The model under review builds one solid part; all positions refer to its coordinate system, in mm. Face numbers are marked on the shaded views. A direction names the side the tool comes from. Round coordinates to 2 decimals unless told otherwise and drop trailing zeros. Loops run counter-clockwise (first coordinate to the right, second up) from the corner with the lowest first, then second, coordinate; pieces in that order, holes last. Notation, with made-up numbers: M 24,2.25 L 51,2.25 A33 cw 51,31.25 Z; hole C 36.25,30 d9. An arc over 180 degrees is marked long. Use a Markdown table: item, result. Add a question column.
```python
from build123d import *

# Parameters (mm, degrees)
SKETCH5_W           = 60
SKETCH5_H           = 55
BOSS_EXTRUDE4_DEPTH = 20
SKETCH6_W           = 55
SKETCH6_H           = 50
CUT_EXTRUDE2_DEPTH  = 17.5
FILLET1_R           = 5
SKETCH8_W           = 45
SKETCH8_H           = 45
BOSS_EXTRUDE5_DEPTH = 5
CUT_EXTRUDE4_REACH  = 49.762
SKETCH9_W           = 15
SKETCH9_H           = 20
CUT_EXTRUDE5_REACH  = 68.802
SKETCH11_W          = 10
SKETCH11_H          = 4


with BuildPart() as part:
    # Sketch5 → Boss-Extrude4 (new body)
    with BuildSketch(Plane(origin=(0, 0, 0), x_dir=(1, 0, 0), z_dir=(0, 1, 0))):
        Rectangle(SKETCH5_W, SKETCH5_H)
    extrude(amount=BOSS_EXTRUDE4_DEPTH)

    # Sketch6 → Cut-Extrude2 (cut)
    with BuildSketch(Plane(origin=(0, 20, 0), x_dir=(1, 0, 0), z_dir=(0, 1, 0))):
        Rectangle(SKETCH6_W, SKETCH6_H)
    extrude(amount=-CUT_EXTRUDE2_DEPTH, mode=Mode.SUBTRACT)

    # Fillet1
    fillet1_edges = [part.edges().sort_by_distance(p)[0] for p in [
        (-30, 10, -27.5),
        (30, 10, -27.5),
        (30, 10, 27.5),
        (-30, 10, 27.5),
    ]]
    fillet(fillet1_edges, radius=FILLET1_R)

    # Sketch8 → Boss-Extrude5 (add)
    with BuildSketch(Plane.XZ):
        Rectangle(SKETCH8_W, SKETCH8_H)
    extrude(amount=BOSS_EXTRUDE5_DEPTH)

    # Sketch9 → Cut-Extrude4 (cut, up to next)
    with BuildSketch(Plane.XZ.offset(5), mode=Mode.PRIVATE) as cut_extrude4_sk1:
        with Locations((-12.5, 10)):
            Rectangle(SKETCH9_W, SKETCH9_H)
    cut_extrude4_tool1 = extrude(cut_extrude4_sk1.sketch, amount=-CUT_EXTRUDE4_REACH, mode=Mode.PRIVATE) & part.part
    add(cut_extrude4_tool1.solids().sort_by_distance((-12.5, -5, 10))[0], mode=Mode.SUBTRACT)

    # Sketch11 → Cut-Extrude5 (cut, up to next)
    with BuildSketch(Plane(origin=(-27.5, 0, 0), x_dir=(0, 0, -1), z_dir=(1, 0, 0)), mode=Mode.PRIVATE) as cut_extrude5_sk1:
        with Locations((0, 14.5)):
            Rectangle(SKETCH11_W, SKETCH11_H)
    cut_extrude5_tool1 = extrude(cut_extrude5_sk1.sketch, amount=-CUT_EXTRUDE5_REACH, mode=Mode.PRIVATE) & part.part
    add(cut_extrude5_tool1.solids().sort_by_distance((-27.5, 14.5, 0))[0], mode=Mode.SUBTRACT)


solid = part.part
```
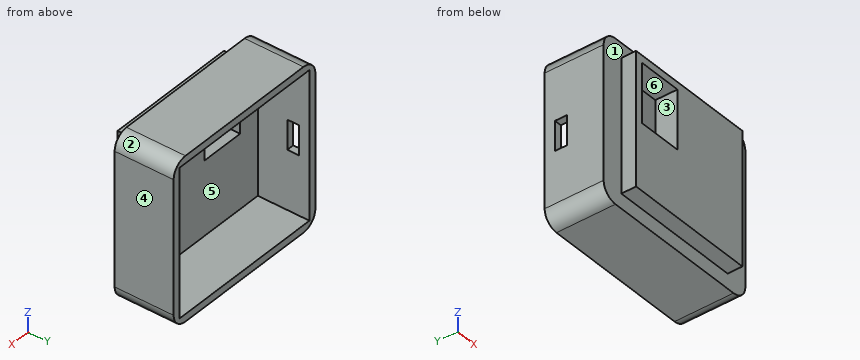
(1) For the marked faces 4, 5 and 6, list the 3-axis set-ups (+Z, -Z, +X, -X, +Y, -Y) from which the entire face can be reached by the end or side of a thin tool; tool diameter is ignored.
(2) Consider section B-B, the plane y = 18. Give the boundary of the cut face in (x, z).
(3) Consider section C-C, the plane z = 12. Give the boundary of the cut face in (x, y).
(4) Consider section D-D, the plane z = -12. Give the boundary of the cut face in (x, y).
(5) Draft analysis for pull direction X (two halves, no side actions). For the marked faces 1, 2 and 3, state which applies: released by +X, released by -X, zero draft, split by the parting line, or undercut.
(6) To check wall thickness, follow probe 1 along Z at (x, y) = (9, 18.75); probe 2 along X at (y, z) = (2.75, 16.5); probe 3 along Z at (x, y) = (-9.5, -2). State the ranges of each line that lie inside material, in increasing order.
(7) Insertion check: pin 1 Ø0.8 at (x, y) = (-29, 15) entering from -Z; pin 2 Ø1.2 at (x, y) = (-28.5, 15) entering from +Z; pin 3 Ø1.5 at (x, y) = (-1, -2.5) entering from -Z. Each pin has a flat end and moves straight along its axis. Give the tip position at first contact, or say it passes through.
(8) Consider section A-A, the plane x = -16. Give the boundary of the cut face in (y, z), then the cut area to 3 significant figures.
Found:
| question | item | result |
|---|---|---|
| 1 | face 4 | +Z, -Z, +X, +Y, -Y |
| 1 | face 5 | +Y |
| 1 | face 6 | +Y, -Y |
| 2 | outline | M -30,-22.5 A5 ccw -25,-27.5 L 25,-27.5 A5 ccw 30,-22.5 L 30,22.5 A5 ccw 25,27.5 L -25,27.5 A5 ccw -30,22.5 Z; hole M -27.5,-25 L 27.5,-25 L 27.5,25 L -27.5,25 Z |
| 3 | outline | M -30,0 L -22.5,0 L -22.5,-5 L -20,-5 L -20,2.5 L -27.5,2.5 L -27.5,20 L -30,20 Z; M -5,-5 L 22.5,-5 L 22.5,0 L 30,0 L 30,20 L 27.5,20 L 27.5,2.5 L -5,2.5 Z |
| 4 | outline | M -30,0 L -22.5,0 L -22.5,-5 L 22.5,-5 L 22.5,0 L 30,0 L 30,20 L 27.5,20 L 27.5,2.5 L -27.5,2.5 L -27.5,20 L -30,20 Z |
| 5 | face 1 | zero draft |
| 5 | face 2 | released by +X |
| 5 | face 3 | undercut |
| 6 | probe 1 | z = -27.5 to -25, 25 to 27.5 |
| 6 | probe 2 | x = -30 to -27.5, 27.5 to 30 |
| 6 | probe 3 | z = -22.5 to 0, 20 to 22.5 |
| 7 | pin 1 | stops at z = -25.97 |
| 7 | pin 2 | stops at z = 26.57 |
| 7 | pin 3 | stops at z = -22.5 |
| 8 | outline | M -5,-22.5 L 0,-22.5 L 0,-27.5 L 20,-27.5 L 20,-25 L 2.5,-25 L 2.5,0 L -5,0 Z; M -5,20 L 2.5,20 L 2.5,25 L 20,25 L 20,27.5 L 0,27.5 L 0,22.5 L -5,22.5 Z |
| 8 | area | 300 mm^2 |
